from build123d import *

# Parameters (mm, degrees)
SKETCH1_R           = 12.7
BOSS_EXTRUDE1_DEPTH = 69.85
CUT_EXTRUDE1_DEPTH  = 10
SKETCH3_R           = 3.571999968
CUT_EXTRUDE2_DEPTH  = 34.925
SKETCH5_R           = 14.7
SKETCH5_R_2         = 3.572
BOSS_EXTRUDE2_DEPTH = 2
BOSS_EXTRUDE5_START = 69.85
SKETCH8_R           = 14.7
BOSS_EXTRUDE5_DEPTH = 2


with BuildPart() as part:
    # Sketch1 → Boss-Extrude1 (new body)
    with BuildSketch(Plane.XY):
        Circle(SKETCH1_R)
    extrude(amount=BOSS_EXTRUDE1_DEPTH)

    # Sketch2 → Cut-Extrude1 (cut)
    with BuildSketch(Plane.XY.offset(69.85)):
        with BuildLine():
            Line((-0.968245837, 1.75), (0.968245837, 1.75))
            ThreePointArc((0.968245837, 1.75), (0, -2), (-0.968245837, 1.75))
        make_face()
    extrude(amount=-CUT_EXTRUDE1_DEPTH, mode=Mode.SUBTRACT)

    # Sketch3 → Cut-Extrude2 (cut)
    with BuildSketch(Plane(origin=(0, 0, 0), x_dir=(-1, 0, 0), z_dir=(0, 0, -1))):
        Circle(SKETCH3_R)
    extrude(amount=-CUT_EXTRUDE2_DEPTH, mode=Mode.SUBTRACT)

    # Sketch5 → Boss-Extrude2 (add)
    with BuildSketch(Plane.XY):
        Circle(SKETCH5_R)
        with Locations(Location((0, 0, 0), (0, 0, 180))):
            Circle(SKETCH5_R_2, mode=Mode.SUBTRACT)
    extrude(amount=BOSS_EXTRUDE2_DEPTH)

    # Sketch8 → Boss-Extrude5 (add)
    with BuildSketch(Plane.XY.offset(BOSS_EXTRUDE5_START)):
        Circle(SKETCH8_R)
        with BuildLine():
            Line((-0.968245837, 1.75), (0.968245837, 1.75))
            ThreePointArc((0.968245837, 1.75), (0, -2), (-0.968245837, 1.75))
        make_face(mode=Mode.SUBTRACT)
    extrude(amount=-BOSS_EXTRUDE5_DEPTH)


solid = part.part
Geometry: final body of the model. Coordinates: model frame, mm. A direction names the side the tool comes from. Coordinates: 2 decimals unless noted, no trailing zeros. Order: outer loops, then holes, each group sorted by start corner. A loop starts at its lowest first (then second) coordinate and runs counter-clockwise, first axis right, second up.
1) Section B-B (y = 0). Return loops of the section in (x, z) (3 decimals).
Result sheet:
outline: (-14.7, 0) - (-3.572, 0) - (-3.572, 34.925) - (3.572, 34.925) - (3.572, 0) - (14.7, 0) - (14.7, 2) - (12.7, 2) - (12.7, 67.85) - (14.7, 67.85) - (14.7, 69.85) - (2, 69.85) - (2, 59.85) - (-2, 59.85) - (-2, 69.85) - (-14.7, 69.85) - (-14.7, 67.85) - (-12.7, 67.85) - (-12.7, 2) - (-14.7, 2) - close
2) Ray query, probe 1 along Z at (x, y) = (-12, 4.5); probe 2 along Y at (x, z) = (0, 24.5); probe 3 along Y at (x, z) = (0, 66.75). Return the intervals inside material, ascending.
Result sheet:
probe 1: z = 0 to 2, 67.85 to 69.85
probe 2: y = -12.7 to -3.57, 3.57 to 12.7
probe 3: y = -12.7 to -2, 1.75 to 12.7
3) Section D-D (z = 55.5). Return loops of the section in (x, y), then the cut area to 3 significant figures.
Result sheet:
outline: circle Ø25.4 at (0, 0)
area: 507 mm2
4) First-contact query: P1, Ø1.9, axis at x = -1, y = 0, coming from the +Z side; P2, Ø3, axis at y = -10.5, z = 33.5, coming from the +X side; P3, Ø2, axis at y = 7, z = 56.5, coming from the -X side. Flat tips, straight axial feed; report the tip coordinate or a pass-through.
Result sheet:
P1: stops at z = 59.85
P2: stops at x = 8.96
P3: stops at x = -11.19
5) Section A-A (x = 0). Return loops of the section in (y, z) (3 decimals), then the cut area to 3 significant figures.
Result sheet:
outline: (-14.7, 0) - (-3.572, 0) - (-3.572, 34.925) - (3.572, 34.925) - (3.572, 0) - (14.7, 0) - (14.7, 2) - (12.7, 2) - (12.7, 67.85) - (14.7, 67.85) - (14.7, 69.85) - (1.75, 69.85) - (1.75, 59.85) - (-2, 59.85) - (-2, 69.85) - (-14.7, 69.85) - (-14.7, 67.85) - (-12.7, 67.85) - (-12.7, 2) - (-14.7, 2) - close
area: 1,500 mm2
6) Section C-C (z = 14.5). Return loops of the section in (x, y), then the cut area to 3 significant figures.
Result sheet:
outline: circle Ø25.4 at (0, 0); hole circle Ø7.14 at (0, 0)
area: 467 mm2
7) Draft query along X for faces 5 (the cylindrical face through (-3.19, -14.35, 0.99)), 6 (the flat face through (-13, 0, 2)), 7 (the flat face through (0, 0, 34.925)). Return one class per face: released by +X, released by -X, zero draft, split by the parting line, or undercut.
Result sheet:
face 5: split by the parting line
face 6: zero draft
face 7: undercut
8) Set-up query: faces 1 (the cylindrical face through (-1.92, 3.01, 17.22)), 2 (the cylindrical face through (0, -2, 65)), 3 (the flat face through (-13, 0, 67.85)), 4 (the cylindrical face through (-3.19, -14.35, 68.86)). Return all of +Z, -Z, +X, -X, +Y, -Y with unobstructed straight access to the full face (end or side cutting, diameter ignored); none if empty.
Result sheet:
face 1: -Z
face 2: +Z
face 3: none
face 4: +Z, -Z
